Job drawing, mm, ordinate dimensions from the low corner. One solid piece. A direction names the side the tool comes from. Round coordinates to 2 decimals unless told otherwise and drop trailing zeros. Order: outer loops, then holes, each group sorted by start corner. A loop starts at its lowest first (then second) coordinate and runs counter-clockwise, first axis right, second up. Notation, with made-up numbers: (13.5, 79) -> (58.5, 79) arc R14 ccw to (58.5, 83) -> close; hole circle Ø5 at (56, 36.5). An arc over 180 degrees is marked (long way). Return JSON: item names as keys, results as strings. Group by question number.
Q1. Probe line 1 along Z through (x, y) = (12.25, 12); line 2 along X through (y, z) = (11.75, 75.5). List the from-to ranges inside material, lowest first.
Q2. Cut at B-B (x = 12). Write the cut outline in (y, z), then the cut area to 3 significant figures.
Q3. Cut at A-A (y = 12). Write the cut outline in (x, z), then the cut area to 3 significant figures.
Q4. Cut at C-C (z = 61.5). Write the cut outline in (x, y), then the cut area to 3 significant figures.
Q5. Cut at D-D (z = 102). Write the cut outline in (x, y).
Q6. Which spindle directions (+Z, -Z, +X, -X, +Y, -Y) get a long thin tool onto all of the face, cutting with end or side? Do the marked faces 1 and 2. Say none if no direction does.
Q7. Flat gauge pins, fed straight in: pin 1 (3 mm diameter, centred on x = 12.5, z = 49, fed in from +Y); pin 2 (5 mm diameter, centred on x = 6.5, z = 94.5, fed in from -Y); pin 3 (1.5 mm diameter, centred on y = 5, z = 51.5, fed in from -X). Where does each tip first touch, or does it go through?
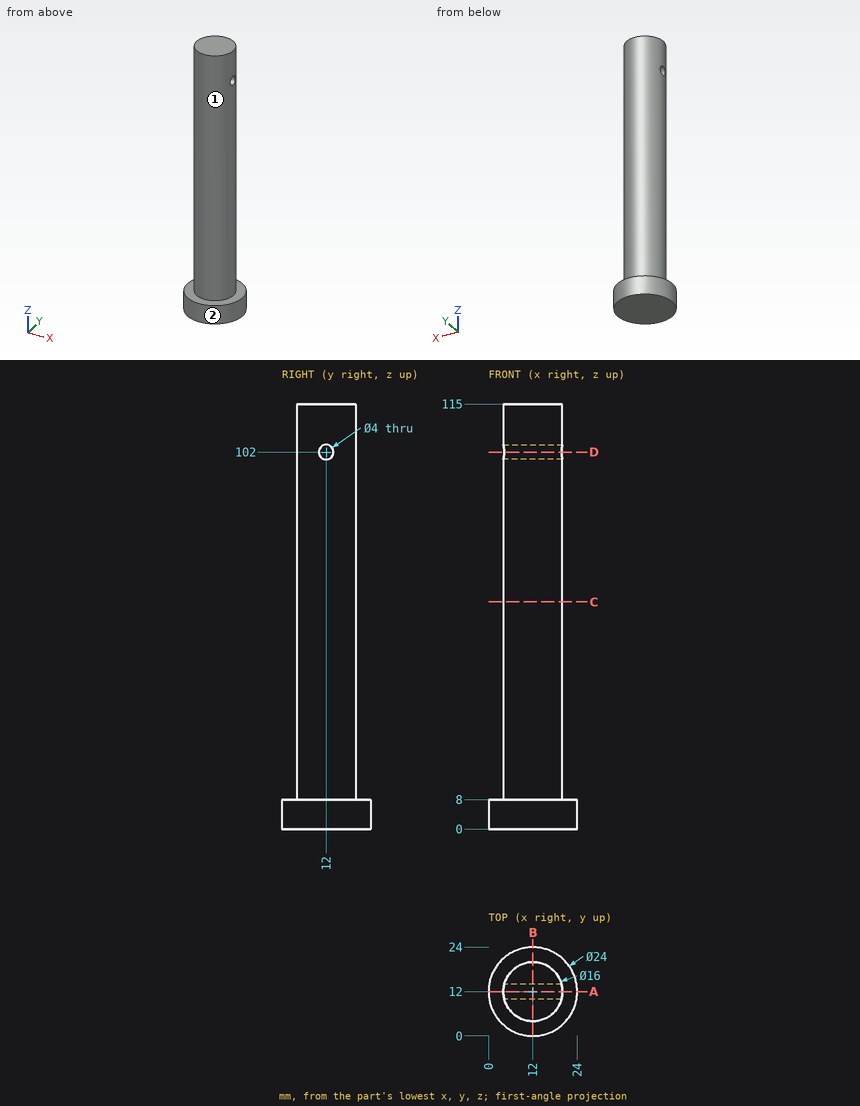
Solution:
{
 "1": {"line 1": "z = 0 to 100, 104 to 115", "line 2": "x = 4 to 20"},
 "2": {"outline": "(0, 0) -> (24, 0) -> (24, 8) -> (20, 8) -> (20, 115) -> (4, 115) -> (4, 8) -> (0, 8) -> close; hole circle Ø4 at (12, 102)", "area": "1,890 mm²"},
 "3": {"outline": "(0, 0) -> (24, 0) -> (24, 8) -> (20, 8) -> (20, 100) -> (4, 100) -> (4, 8) -> (0, 8) -> close; (4, 104) -> (20, 104) -> (20, 115) -> (4, 115) -> close", "area": "1,840 mm²"},
 "4": {"outline": "circle Ø16 at (12, 12)", "area": "201 mm²"},
 "5": {"outline": "(4.25, 10) arc R8 ccw to (19.75, 10) -> close; (4.25, 14) -> (19.75, 14) arc R8 ccw to start"},
 "6": {"face 1": "+Z", "face 2": "+Z, -Z"},
 "7": {"pin 1": "stops at y = 20", "pin 2": "stops at y = 4.58", "pin 3": "stops at x = 7.01"}
}
